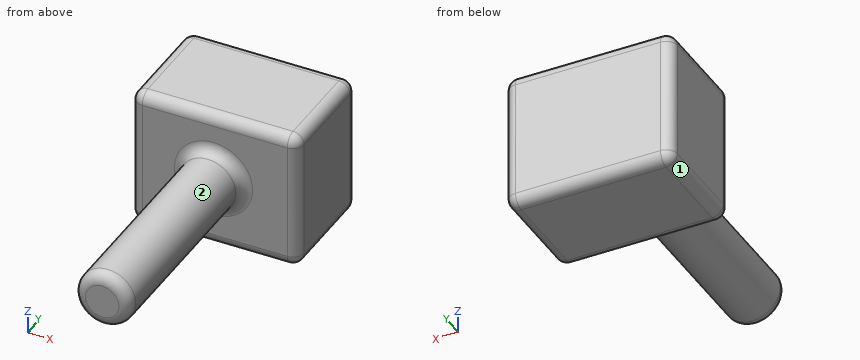
from build123d import *

# Parameters (mm, degrees)
F0_W     = 76.2
F0_H     = 63.5
F1_DEPTH = 50.546
F2_R     = 12.7
F3_DEPTH = 98.298
F4_R     = 5.08
F5_R     = 5.08
F6_R     = 5.08


with BuildPart() as f1:
    # F0 (on Front) → F1 (new body)
    with BuildSketch(Plane.XZ):
        with Locations((-38.1, 31.75)):
            Rectangle(F0_W, F0_H)
    extrude(amount=F1_DEPTH)

    # F2 (on face) → F3 (join)
    with BuildSketch(Plane.XZ.offset(50.546)):
        with Locations((-38.666781, 32.61992)):
            Circle(F2_R)
    extrude(amount=F3_DEPTH)

    # F4
    f4_edges = [f1.edges().sort_by_distance(p)[0] for p in [
        (0, -25.273, 0),
        (0, -25.273, 63.5),
        (-76.2, -25.273, 63.5),
        (-76.2, -25.273, 0),
    ]]
    fillet(f4_edges, radius=F4_R)

    # F5
    f5_edges = [f1.edges().sort_by_distance(p)[0] for p in [
        (-38.1, -50.546, 0),
        (-38.1, 0, 0),
    ]]
    fillet(f5_edges, radius=F5_R)

    # F6
    f6_edges = [f1.edges().sort_by_distance(p)[0] for p in [
        (-25.966781, -99.695, 32.61992),
        (-51.366781, -50.546, 32.61992),
        (-51.366781, -148.844, 32.61992),
    ]]
    fillet(f6_edges, radius=F6_R)


solid = f1.part
The model under review builds one solid part; all positions refer to its coordinate system, in mm. Face numbers are marked on the shaded views. A direction names the side the tool comes from. Give positions to 0.01 mm unless a question says otherwise; leave off trailing zeros. Order: outer loops, then holes, each group sorted by start corner. A loop starts at its lowest first (then second) coordinate and runs counter-clockwise, first axis right, second up. Notation, with made-up numbers: (-3.5, -15) -> (2.5, -15) arc R30 ccw to (2.5, 18) -> close; hole circle Ø2 at (56.25, 1). An arc over 180 degrees is marked (long way). Write item = value, one per line. Start each with the question number.
(1) For L1, parallel to Y at x = -57, z = 55; L2, parallel to X at y = -69, z = 41; L3, parallel to X at y = -76, z = 27, list the stretches that pass through material, from the lowest coordinate up. Write a range as from..to.
(2) For pin 1 Ø4 at (x, z) = (-16.5, 56.5) entering from -Y; pin 2 Ø12 at (x, y) = (-53.5, -78) entering from +Z; pin 3 Ø2 at (y, z) = (-64.5, 30.5) entering from -X, all flat-tipped, find the tip position at first contact; note any pin that passes through.
(3) Take a section at C-C (y = -120). Write out the cut boundary in (x, z), plus the area to 3 significant figures.
(4) Take a section at B-B (z = 52). Write out the cut boundary in (x, y), plus the area to 3 significant figures.
(5) Take a section at A-A (x = -61). Write out the cut boundary in (y, z), plus the area to 3 significant figures.
(6) Tool access review of the marked faces 1 and 2: name each direction out of +Z, -Z, +X, -X, +Y, -Y from which nothing blocks a thin tool from reaching the whole face with its end or side.
Returned:
q1.L1 = -50.55..0
q1.L2 = -48.21..-29.12
q1.L3 = -50.06..-27.28
q2.pin_1 = -50.55
q2.pin_2 = 41.74
q2.pin_3 = -51.32
q3.outline = circle Ø25.4 at (-38.67, 32.62)
q3.area = 507 mm²
q4.outline = (-76.2, -45.47) arc R5.08 ccw to (-71.12, -50.55) -> (-5.08, -50.55) arc R5.08 ccw to (0, -45.47) -> (0, -5.08) arc R5.08 ccw to (-5.08, 0) -> (-71.12, 0) arc R5.08 ccw to (-76.2, -5.08) -> close
q4.area = 3,830 mm²
q5.outline = (-50.55, 5.08) arc R5.08 ccw to (-45.47, 0) -> (-5.08, 0) arc R5.08 ccw to (0, 5.08) -> (0, 58.42) arc R5.08 ccw to (-5.08, 63.5) -> (-45.47, 63.5) arc R5.08 ccw to (-50.55, 58.42) -> close
q5.area = 3,190 mm²
q6.face_1 = -Z, -X, +Y, -Y
q6.face_2 = -Y
